Print and shaded views of the part. All mm, measured from the part's lowest x, y and z. A direction names the side the tool comes from. Coordinates: 2 decimals unless noted, no trailing zeros. Write each loop counter-clockwise with the first axis right and the second up, starting at its lowest first coordinate (ties: lowest second). Pieces come first, ordered by that corner, then holes. Notation, with made-up numbers: (77.25, 33.5) -> (85.25, 33.5) arc R24 cw to (85.25, 64.5) -> close; hole circle Ø7 at (48, 6). An arc over 180 degrees is marked (long way). Write item = value, one per line.
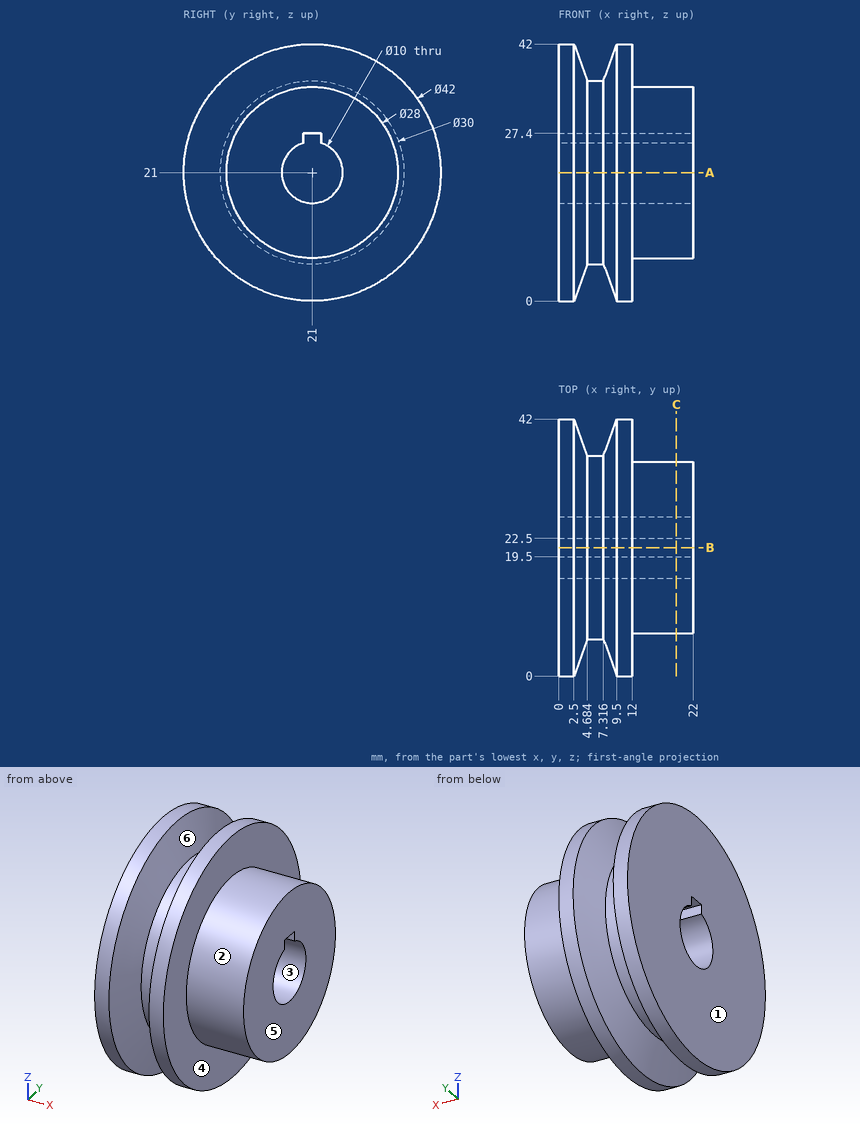
Q1. Saw through at B-B on y = 21. Give the cut face in (x, z).
Model answer:
outline = (0, 0) -> (2.5, 0) -> (4.68, 6) -> (7.32, 6) -> (9.5, 0) -> (12, 0) -> (12, 7) -> (22, 7) -> (22, 16) -> (0, 16) -> close; (0, 27.4) -> (22, 27.4) -> (22, 35) -> (12, 35) -> (12, 42) -> (9.5, 42) -> (7.32, 36) -> (4.68, 36) -> (2.5, 42) -> (0, 42) -> close
Q2. Probe line 1 (Y direction, x = 11.75, z = 21); line 2 (Y direction, x = 6.75, z = 21); line 3 (X direction, y = 34, z = 15). List the from-to ranges inside material, lowest first. Write a range as from..to.
Model answer:
line_1 = 0..16, 26..42
line_2 = 6..16, 26..36
line_3 = 0..12
Q3. Pin check, flat tips, straight feed: pin 1 (11.5 mm diameter, centred on y = 21, z = 21, fed in from +X); pin 2 (10 mm diameter, centred on x = 19, z = 27, fed in from +Y); pin 3 (2 mm diameter, centred on x = 16, y = 14, fed in from +Z); pin 4 (0.8 mm diameter, centred on x = 6.5, z = 26.5, fed in from +Y). Stop position of each tip, or through.
Model answer:
pin_1 = 22
pin_2 = 34.96
pin_3 = 33.65
pin_4 = 35.11
Q4. Saw through at A-A on z = 21. Give the cut face in (x, y), and give its area (3 significant figures).
Model answer:
outline = (0, 0) -> (2.5, 0) -> (4.68, 6) -> (7.32, 6) -> (9.5, 0) -> (12, 0) -> (12, 7) -> (22, 7) -> (22, 16) -> (0, 16) -> close; (0, 26) -> (22, 26) -> (22, 35) -> (12, 35) -> (12, 42) -> (9.5, 42) -> (7.32, 36) -> (4.68, 36) -> (2.5, 42) -> (0, 42) -> close
area = 506 mm²
Q5. Saw through at C-C on x = 19.25. Give the cut face in (y, z), and give its area (3 significant figures).
Model answer:
outline = circle Ø28 at (21, 21); hole (19.5, 25.77) arc R5 ccw (long way) to (22.5, 25.77) -> (22.5, 27.4) -> (19.5, 27.4) -> close
area = 533 mm²
Q6. Which spindle directions (+Z, -Z, +X, -X, +Y, -Y) get a long thin tool onto all of the face, cutting with end or side? Do the marked faces 4, 5 and 6. Say none if no direction does.
Model answer:
face_4 = +X
face_5 = +Z, -Z, +X, +Y, -Y
face_6 = none
Q7. Mould opens along Z. For the marked faces 1, 2 and 3 say: released by +Z, released by -Z, zero draft, split by the parting line, or undercut.
Model answer:
face_1 = zero draft
face_2 = split by the parting line
face_3 = undercut
